```python
from build123d import *

# Parameters (mm, degrees)
SKETCH1_W           = 50
SKETCH1_H           = 40
BOSS_EXTRUDE1_DEPTH = 10
SKETCH2_W           = 20
SKETCH2_H           = 40
BOSS_EXTRUDE2_DEPTH = 20
CUT_EXTRUDE1_DEPTH  = 20
CUT_EXTRUDE5_DEPTH  = 20


with BuildPart() as part:
    # Sketch1 → Boss-Extrude1 (new body)
    with BuildSketch(Plane(origin=(0, 0, 0), x_dir=(1, 0, 0), z_dir=(0, 1, 0))):
        Rectangle(SKETCH1_W, SKETCH1_H)
    extrude(amount=BOSS_EXTRUDE1_DEPTH)

    # Sketch2 → Boss-Extrude2 (add)
    with BuildSketch(Plane(origin=(0, 10, 0), x_dir=(1, 0, 0), z_dir=(0, 1, 0))):
        with Locations((-15, 0)):
            Rectangle(SKETCH2_W, SKETCH2_H)
    extrude(amount=BOSS_EXTRUDE2_DEPTH)

    # Sketch3 → Cut-Extrude1 (cut)
    with BuildSketch(Plane(origin=(-5, 0, 0), x_dir=(0, 0, -1), z_dir=(1, 0, 0))):
        Polygon((20, 30), (-20, 10), (-20, 30), align=None)
    extrude(amount=-CUT_EXTRUDE1_DEPTH, mode=Mode.SUBTRACT)

    # Sketch5 → Cut-Extrude5 (cut)
    with BuildSketch(Plane.XY.offset(20)):
        Polygon((0, 10), (25, 0), (25, 10), align=None)
    extrude(amount=-CUT_EXTRUDE5_DEPTH, mode=Mode.SUBTRACT)


solid = part.part
```
Part model, mm, in its own coordinate system. A direction names the side the tool comes from. Give positions to 0.01 mm unless a question says otherwise; leave off trailing zeros. Order: outer loops, then holes, each group sorted by start corner. A loop starts at its lowest first (then second) coordinate and runs counter-clockwise, first axis right, second up. Notation, with made-up numbers: M -7.5,77 L 5.5,77 A18 ccw 5.5,82 Z; hole C 62.25,31.25 d3. An arc over 180 degrees is marked long. Use a Markdown table: item, result. Add a question column.
(1) Saw through at C-C, the plane y = 25.5. Give the cut face in (x, z).
(2) Saw through at D-D, the plane x = -6.5. Give the cut face in (y, z).
(3) Saw through at B-B, the plane x = 4. Give the cut face in (y, z).
(4) Probe line 1 along Y through (x, z) = (10.5, -4); line 2 along X through (y, z) = (13, 8); line 3 along Z through (x, y) = (19, 5.75). List the from-to ranges inside material, lowest first. Write a range as [from, to].
(5) Saw through at A-A, the plane z = 11. Give the cut face in (x, y), and give its area (3 significant figures).
(6) 3-axis set-ups, long thin cutter, end or side, ignore diameter. For faces 1 (the face through (6, 10, -5)), 2 (the face through (12.32, 5.07, 10.14)), 3 (the face through (-15, 20, 0)): which of +Z, -Z, +X, -X, +Y, -Y reach the whole face in a straight line?
(7) Drop flat-ended pins along their axis: P1, Ø6, axis at x = 0.5, z = -14.5, coming from the +Y side; P2, Ø1, axis at x = 12.5, z = 9.5, coming from the +Y side; P3, Ø1.5, axis at y = 18, z = 8, coming from the -X side. Give the stop position or say it passes through.
Answer key:
| question | item | result |
|---|---|---|
| 1 | outline | M -25,-20 L -5,-20 L -5,-11 L -25,-11 Z |
| 2 | outline | M 0,-20 L 30,-20 L 10,20 L 0,20 Z |
| 3 | outline | M 0,-20 L 10,-20 L 10,0 L 8.4,0 L 8.4,20 L 0,20 Z |
| 4 | line 1 | [0, 10] |
| 4 | line 2 | [-25, -5] |
| 4 | line 3 | [-20, 0] |
| 5 | outline | M -25,0 L 25,0 L 0,10 L -5,10 L -5,14.5 L -25,14.5 Z |
| 5 | area | 465 mm^2 |
| 6 | face 1 | +Z, -Z, +X, +Y |
| 6 | face 2 | +Z, +X, +Y |
| 6 | face 3 | +Z, +X, -X, +Y |
| 7 | P1 | y = 10 |
| 7 | P2 | y = 5.2 |
| 7 | P3 | through |
